Autodesk Inventor part; units mm, degrees
ref_plane "YZ Plane" through (0, 0, 0) normal (1, 0, 0) x (0, 1, 0)
ref_plane "XZ Plane" through (0, 0, 0) normal (0, 1, 0) x (-1, 0, 0)
ref_plane "XY Plane" through (0, 0, 0) normal (0, 0, 1) x (1, 0, 0)
sketch "Sketch1" plane through (0, 0, 0) normal (0, 1, 0) x (-1, 0, 0)
  arc A0 (90.3834, -85.781) -> (90.3834, -67.2115) centre (86.6694, -76.4962) ccw
  arc A1 (40.3834, -47.2115) -> (26.6694, -56.4962) centre (36.6694, -56.4962) ccw
  arc A2 (26.6694, -96.4962) -> (40.3834, -105.781) centre (36.6694, -96.4962) ccw
  line L0 (40.3834, -47.2115) -> (90.3834, -67.2115)
  line L1 (90.3834, -85.781) -> (40.3834, -105.781)
  circle A3 centre (86.6694, -76.4962) radius 5
  circle A4 centre (36.6694, -56.4962) radius 5
  circle A5 centre (36.6694, -96.4962) radius 5
  arc A6 (54.9839, -83.5808) -> (54.6671, -69.8665) centre (64.6694, -76.4962) ccw
  arc A7 (34.6694, -70.7615) -> (34.6706, -82.7615) centre (34.6706, -76.7615) ccw
  line L2 (34.6694, -70.7615) -> (53.0001, -70.7615)
  line L3 (53.3697, -82.7615) -> (34.6706, -82.7615)
  arc A8 (23.7082, -61.243) -> (23.7082, -92.2801) centre (34.6706, -76.7615) ccw
  line L4 (26.6694, -96.4962) -> (26.6694, -97.9974)
  line L5 (26.6694, -55.5256) -> (26.6694, -56.4962)
  arc A9 (23.7082, -61.243) -> (26.6694, -55.5256) centre (19.6694, -55.5256) ccw
  arc A10 (26.6694, -97.9974) -> (23.7082, -92.2801) centre (19.6694, -97.9974) ccw
  arc A11 (53.0001, -70.7615) -> (54.6671, -69.8665) centre (53.0001, -68.7615) ccw
  arc A12 (54.9839, -83.5808) -> (53.3697, -82.7615) centre (53.3697, -84.7615) ccw
  point P0 (0, 0)
  point P1 (54.4349, -82.7615)
  point P2 (54.1284, -70.7615)
  point P3 (26.6694, -59.5284)
  point P4 (26.6694, -93.9947)
  dimension "d0" = 50
  dimension "d1" = 0
  dimension "d2" = 20
  dimension "d3" = 20
  dimension "d4" = 20
  dimension "d5" = 40
  dimension "d6" = 20
  dimension "d7" = 10
  dimension "d8" = 10
  dimension "d9" = 10
  dimension "d10" = 12
  dimension "d11" = 30
  dimension "d12" = 6
  dimension "d13" = 0
  dimension "d14" = 22
  dimension "d16" = 7
  dimension "d17" = 7
  dimension "d18" = 2
extrude "Extrusion1" add sketch "Sketch1" along normal blind 10
equation "\"d3\" = d2"
equation "\"d4\" = d2"
equation "\"d6\" = 0.5 * d5"
equation "\"d8\" = d7"
equation "\"d9\" = d7"
For this review, take the finished solid that the model builds, in its own axes (mm). A direction names the side the tool comes from. Coordinates: 2 decimals unless noted, no trailing zeros. Write each loop counter-clockwise with the first axis right and the second up, starting at its lowest first coordinate (ties: lowest second). Pieces come first, ordered by that corner, then holes.
(1) Add section A-A on z = -93.5. Give the boundary of the cut face in (x, y).
(2) For pin 1 Ø13 at (x, z) = (-36.67, -56.5) entering from -Y; pin 2 Ø8 at (x, z) = (-36.67, -96.5) entering from +Y; pin 3 Ø2 at (y, z) = (5.5, -79.5) entering from -X; pin 4 Ø5 at (x, y) = (-42, 3.5) entering from +Z, all flat-tipped, find the tip position at first contact; note any pin that passes through.
(3) Add section B-B on x = -89.5. Give the boundary of the cut face in (y, z).
(4) Wall thickness on probe 1 along X at (y, z) = (5.75, -78); probe 2 along Z at (x, y) = (-36, 1.75); probe 3 along X at (y, z) = (4.5, -72.5): over which ranges is each line inside the solid? List them lowest first.
(5) Tool access review of faces 4 (the face through (-47, 10, -69)), 5 (the face through (-44, 5, -70.762)): name each direction out of +Z, -Z, +X, -X, +Y, -Y from which nothing blocks a thin tool from reaching the whole face with its end or side.
(6) Add section C-C on y = 6.25. Give the boundary of the cut face in (x, z).
(7) The part is to be moulded in two halves that separate along X. For faces 1 (the face through (-44, 5, -82.762)), 2 (the face through (-65.733, 4.93, -95.641)), 3 (the face through (-25.864, 4.93, -94.737)), say which applies: +X half, -X half, draft (parallel to the pull), parting line (faces both ways), or undercut.
(8) Add section D-D on z = -49.5. Give the boundary of the cut face in (x, y), then the cut area to 3 significant figures.
Answer sheet:
1. outline: (-71.09, 0) - (-40.67, 0) - (-40.67, 10) - (-71.09, 10) - close; (-32.67, 0) - (-25.03, 0) - (-25.03, 10) - (-32.67, 10) - close
2. pin 1: stops at y = 0
2. pin 2: passes through
2. pin 3: stops at x = -96.47
2. pin 4: stops at z = -46.91
3. outline: (0, -86.13) - (10, -86.13) - (10, -80.62) - (0, -80.62) - close; (0, -72.37) - (10, -72.37) - (10, -66.86) - (0, -66.86) - close
4. probe 1: x = -96.56 to -91.44, -81.9 to -76.57, -28.8 to -15.71
4. probe 2: z = -106.47 to -101.45, -91.54 to -82.76, -70.76 to -61.45, -51.54 to -46.52
4. probe 3: x = -95.84 to -89.67, -83.66 to -75.98, -30.45 to -16.15
5. face 4: +Z, -Z, +X, -X, +Y
5. face 5: +Y, -Y
6. outline: (-90.38, -85.78) - (-40.38, -105.78) arc R10 ccw to (-26.67, -96.5) - (-26.67, -98) arc R7 cw to (-23.71, -92.28) arc R19 ccw to (-23.71, -61.24) arc R7 cw to (-26.67, -55.53) - (-26.67, -56.5) arc R10 ccw to (-40.38, -47.21) - (-90.38, -67.21) arc R10 ccw to start; hole circle Ø10 at (-86.67, -76.5); hole (-54.98, -83.58) arc R2 cw to (-53.37, -82.76) - (-34.67, -82.76) arc R6 ccw to (-34.67, -70.76) - (-53, -70.76) arc R2 cw to (-54.67, -69.87) arc R12 ccw (long way) to start; hole circle Ø10 at (-36.67, -96.5); hole circle Ø10 at (-36.67, -56.5)
7. face 1: undercut
7. face 2: -X half
7. face 3: +X half
8. outline: (-46.1, 0) - (-29.52, 0) - (-29.52, 10) - (-46.1, 10) - close
8. area: 166 mm2
